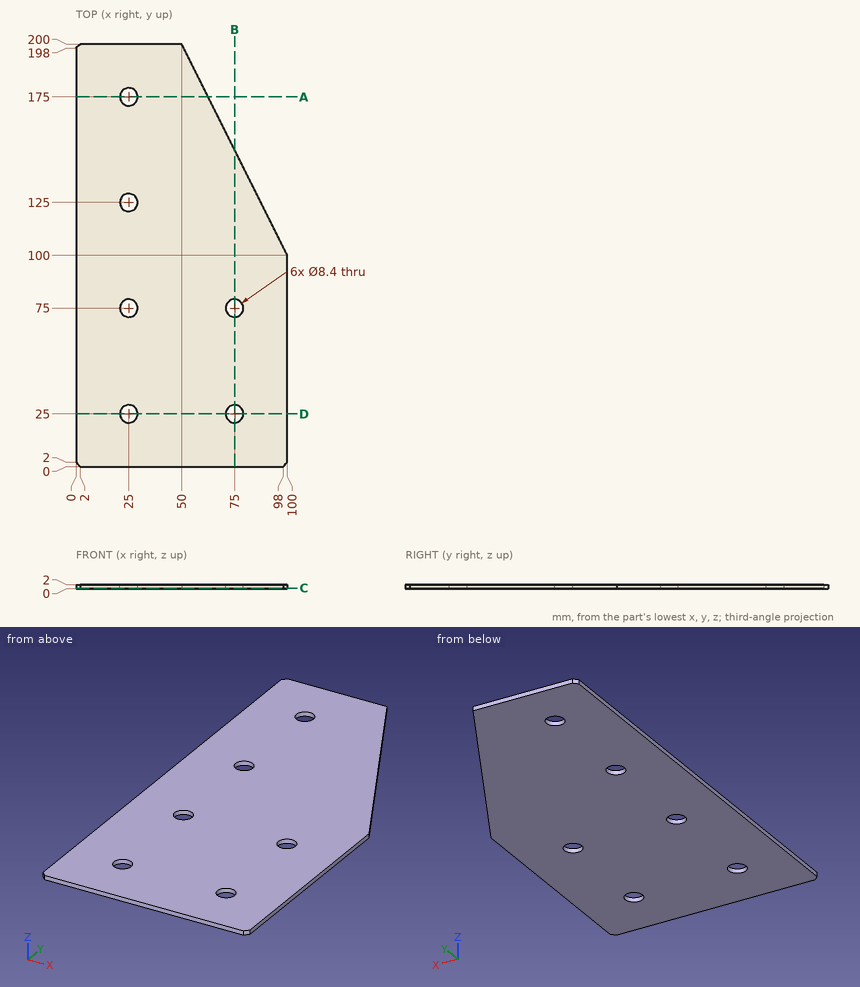
Here's the drawing with two shaded views (mm, measured from the low corner). I have some questions. Round coordinates to 2 decimals unless told otherwise and drop trailing zeros. Order: outer loops, then holes, each group sorted by start corner. A loop starts at its lowest first (then second) coordinate and runs counter-clockwise, first axis right, second up. Notation, with made-up numbers: (-38, 81.5) -> (18, 81.5) arc R30 cw to (18, 115.5) -> close; hole circle Ø6 at (89.25, 89.5). An arc over 180 degrees is marked (long way). Write each question's results on one line, items separated by ' | '. Start each with the question number.
Item 1: Please list where these lines run through material, in increasing order: L1, parallel to Y at x = 25, z = 1.25; L2, parallel to X at y = 75, z = 1.25; L3, parallel to Y at x = 75, z = 0.45.
Item 2: If we section it at C-C, the plane z = 0.4: Write out the boundary of the cut face in (x, y), then the cut area to 3 significant figures.
Item 3: If we section it at B-B, the plane x = 75: Write out the boundary of the cut face in (y, z).
Item 4: If we section it at A-A, the plane y = 175: Write out the boundary of the cut face in (x, z).
Item 5: If we section it at D-D, the plane y = 25: Write out the boundary of the cut face in (x, z), then the cut area to 3 significant figures.
Results:
1) L1: y = 0 to 20.8, 29.2 to 70.8, 79.2 to 120.8, 129.2 to 170.8, 179.2 to 200 | L2: x = 0 to 20.8, 29.2 to 70.8, 79.2 to 100 | L3: y = 0 to 20.8, 29.2 to 70.8, 79.2 to 150
2) outline: (0, 2) -> (2, 0) -> (98, 0) -> (100, 2) -> (100, 100) -> (50, 200) -> (2, 200) -> (0, 198) -> close; hole circle Ø8.4 at (25, 25); hole circle Ø8.4 at (25, 75); hole circle Ø8.4 at (25, 125); hole circle Ø8.4 at (25, 175); hole circle Ø8.4 at (75, 25); hole circle Ø8.4 at (75, 75) | area: 17,200 mm2
3) outline: (0, 0) -> (20.8, 0) -> (20.8, 2) -> (0, 2) -> close; (29.2, 0) -> (70.8, 0) -> (70.8, 2) -> (29.2, 2) -> close; (79.2, 0) -> (150, 0) -> (150, 2) -> (79.2, 2) -> close
4) outline: (0, 0) -> (20.8, 0) -> (20.8, 2) -> (0, 2) -> close; (29.2, 0) -> (62.5, 0) -> (62.5, 2) -> (29.2, 2) -> close
5) outline: (0, 0) -> (20.8, 0) -> (20.8, 2) -> (0, 2) -> close; (29.2, 0) -> (70.8, 0) -> (70.8, 2) -> (29.2, 2) -> close; (79.2, 0) -> (100, 0) -> (100, 2) -> (79.2, 2) -> close | area: 166 mm2
